Geometry: final body of the model. Coordinates: model frame, mm. A direction names the side the tool comes from. Give positions to 0.01 mm unless a question says otherwise; leave off trailing zeros. Write each loop counter-clockwise with the first axis right and the second up, starting at its lowest first coordinate (ties: lowest second). Pieces come first, ordered by that corner, then holes. Notation, with made-up numbers: M 53.25,50.25 L 68.25,50.25 A26 cw 68.25,65.25 Z; hole C 25.5,-5 d9. An arc over 180 degrees is marked long. Answer as a JSON object with one key per item and string values.
from build123d import *

# Parameters (mm, degrees)
F1_DEPTH = 57.912
F2_R     = 5.08
F3_T     = -2.54


# Not quite as in the source:
# - a shell that OpenCascade refuses in one call is made with other operations: the cavity is built on its own and cut out


with BuildPart() as f1:
    # F0 (on Front) → F1 (new body)
    with BuildSketch(Plane.XZ):
        Polygon((-7.2342143664, 44.1616670006), (-40.2542143664, 44.1616670006), (-40.2542143664, 13.6816670006), (-23.2922839558, 13.6816670006), (-23.2922839558, -6.6383329994), (55.4477160442, -6.6383329994), (55.4477160442, 18.7616670006), (-7.2342143664, 28.9216670006), align=None)
    extrude(amount=F1_DEPTH)

    # F2
    f2_edges = [f1.edges().sort_by_distance(p)[0] for p in [
        (-7.234214, -28.956, 44.161667),
        (-7.234214, -28.956, 28.921667),
        (55.447716, -28.956, 18.761667),
        (55.447716, -28.956, -6.638333),
        (-40.254214, -28.956, 44.161667),
        (-40.254214, -28.956, 13.681667),
        (-23.292284, -28.956, 13.681667),
        (-23.292284, -28.956, -6.638333),
    ]]
    fillet(f2_edges, radius=F2_R)

    # F3: a shell. OpenCascade refuses it in one call, so the cavity is built on its own and cut out:
    # the body offset inwards by the wall thickness, plus a prism from it out through each open face.
    f3_core = offset(f1.part, amount=F3_T, mode=Mode.PRIVATE)
    f3_exits = [f3_core.faces().sort_by_distance(p)[0] for p in [
        (52.907716, -28.956, 6.440221),
    ]]
    add(f3_core, mode=Mode.SUBTRACT)
    extrude(f3_exits, amount=-F3_T, mode=Mode.SUBTRACT)


solid = f1.part
1) Cut plane A-A on z = 34.5. Return loops of the section in (x, y), and give its area (3 significant figures).
Geometry check:
{"outline": "M -40.25,-57.91 L -7.23,-57.91 L -7.23,0 L -40.25,0 Z; hole M -37.71,-55.37 L -9.77,-55.37 L -9.77,-2.54 L -37.71,-2.54 Z", "area": "436 mm2"}
2) Contact query for flat-ended pins moving along their axis: P1, Ø6, axis at x = 30.5, y = -36.5, coming from the +Z side; P2, Ø2, axis at x = -31, y = -41.5, coming from the -Z side; P3, Ø2, axis at x = 54, y = -31, coming from the +Z side. Output: stop coordinate, or through.
Geometry check:
{"P1": "stops at z = 23.29", "P2": "stops at z = 13.68", "P3": "stops at z = 18.78"}
3) Cut plane B-B on x = 33. Return loops of the section in (y, z), and give its area (3 significant figures).
Geometry check:
{"outline": "M -57.91,-6.64 L 0,-6.64 L 0,22.4 L -57.91,22.4 Z; hole M -55.37,-4.1 L -2.54,-4.1 L -2.54,19.83 L -55.37,19.83 Z", "area": "418 mm2"}
4) Pull-direction query (Z, two-part tool) for faces 5 (the flat face through (-20.752, -29, 4)), 6 (the cylindrical face through (53.92, -29.36, -5.19)), 7 (the cylindrical face through (-5.99, -29.361, 29.914)); classes: pulls with the +Z half, pulls with the -Z half, needs draft (parallel to the pull), parting line crosses it, or undercut.
Geometry check:
{"face 5": "undercut", "face 6": "pulls with the -Z half", "face 7": "pulls with the +Z half"}
5) Set-up query: faces 1 (the flat face through (54, -29, -1.558)), 2 (the cylindrical face through (-36.95, -29.33, 40.9)), 3 (the flat face through (-32, -29, 13.682)), 4 (the flat face through (-7.234, -29, 36)). Return all of +Z, -Z, +X, -X, +Y, -Y with unobstructed straight access to the full face (end or side cutting, diameter ignored); none if empty.
Geometry check:
{"face 1": "+X", "face 2": "none", "face 3": "-Z, -X, +Y, -Y", "face 4": "+Z, +X, +Y, -Y"}
6) Cut plane C-C on z = 3.5. Return loops of the section in (x, y), and give its area (3 significant figures).
Geometry check:
{"outline": "M -23.29,-57.91 L 55.45,-57.91 L 55.45,-55.37 L -20.75,-55.37 L -20.75,-2.54 L 55.45,-2.54 L 55.45,0 L -23.29,0 Z", "area": "534 mm2"}
7) Line query: line 1 (Y direction, x = -15.5, z = 11.5); line 2 (X direction, y = -9.5, z = 39); line 3 (Z direction, x = -16, y = -10). Output: solid intervals per line, ascending. Write a range as from..to.
Geometry check:
{"line 1": "y = -57.91..-55.37, -2.54..0", "line 2": "x = -40.25..-37.71, -9.77..-7.23", "line 3": "z = -6.64..-4.1, 41.62..44.16"}
